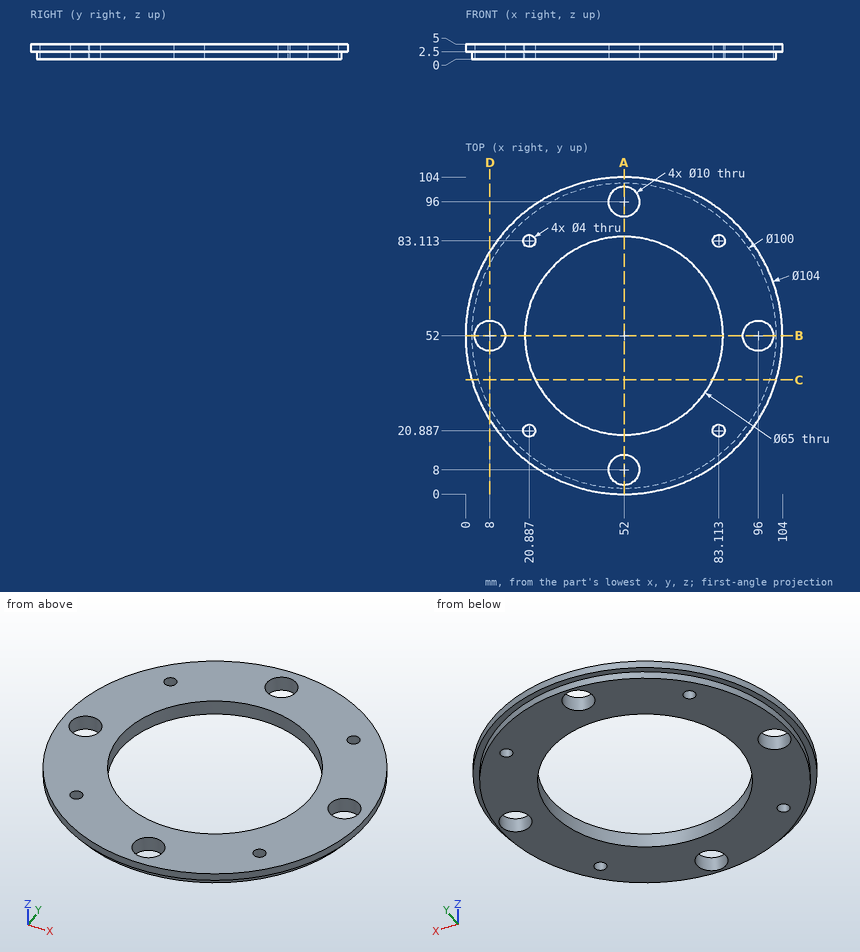
Can you work these out from the drawing? Everything is in mm from the part's minimum corner. Give positions to 0.01 mm unless a question says otherwise; leave off trailing zeros. Loops run counter-clockwise (first coordinate to the right, second up) from the corner with the lowest first, then second, coordinate; pieces in that order, holes last. Notation, with made-up numbers: M 67,33 L 99,33 A16 cw 99,45 Z; hole C 55,-27.75 d3. An arc over 180 degrees is marked long. Use CSV: the item, a comma, the result in double quotes. Start each with the question number.
1. For P1, Ø1.5, axis at x = 27.5, z = 3.5, coming from the +Y side; P2, Ø3, axis at x = 47, z = 4.5, coming from the +Y side; P3, Ø2, axis at x = 85, z = 4.5, coming from the -Y side, each with a flat end and sliding along its axis, tell me the tip position at first contact or that it passes through.
2. Imagine slicing it at D-D, the plane x = 8. Write out the boundary of the cut face in (y, z).
3. Imagine slicing it at C-C, the plane y = 37.5. Write out the boundary of the cut face in (x, z).
4. If I drill on L1, parallel to Y at x = 22.5, z = 2.3 (1 decimal); L2, parallel to Z at x = 6.5, y = 74.5; L3, parallel to X at y = 33, z = 1.05, over which ranges is the centre line in solid material (lowest first)?
5. Imagine slicing it at A-A, the plane x = 52. Write out the boundary of the cut face in (y, z), plus the area to 3 significant figures.
Response values:
1,P1,"y = 98.26"
1,P2,"y = 103.88"
1,P3,"y = 11.01"
2,outline,"M 24.29,2.5 L 28.25,2.5 L 28.25,0 L 47,0 L 47,5 L 24.29,5 Z; M 57,0 L 75.75,0 L 75.75,2.5 L 79.71,2.5 L 79.71,5 L 57,5 Z"
3,outline,"M 2.06,2.5 L 4.15,2.5 L 4.15,0 L 22.91,0 L 22.91,5 L 2.06,5 Z; M 81.09,0 L 99.85,0 L 99.85,2.5 L 101.94,2.5 L 101.94,5 L 81.09,5 Z"
4,L1,"11.6 to 19.7, 22.1 to 38.4, 65.6 to 81.9, 84.3 to 92.4"
4,L2,"2.5 to 5"
4,L3,"5.75 to 25.63, 78.37 to 98.25"
5,outline,"M 0,2.5 L 2,2.5 L 2,0 L 3,0 L 3,5 L 0,5 Z; M 13,0 L 19.5,0 L 19.5,5 L 13,5 Z; M 84.5,0 L 91,0 L 91,5 L 84.5,5 Z; M 101,0 L 102,0 L 102,2.5 L 104,2.5 L 104,5 L 101,5 Z"
5,area,"85.0 mm^2"
